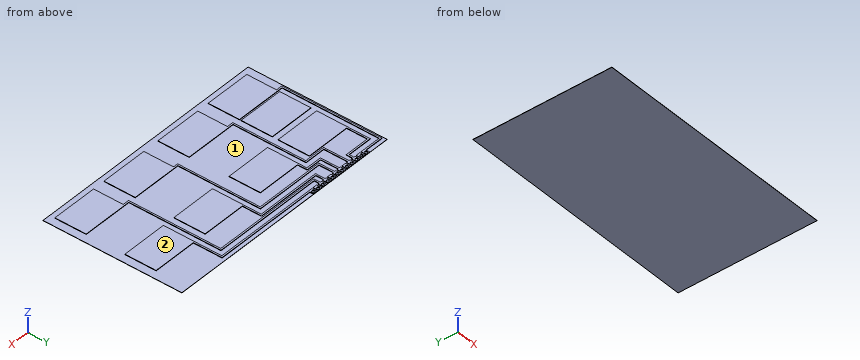
from build123d import *

# Parameters (mm, degrees)
F0_W     = 308
F0_H     = 174
F1_DEPTH = 0.25
F2_R     = 1.6
F2_W     = 57.88946
F2_H     = 39.180715
F3_DEPTH = 0.5


with BuildPart() as f1:
    # F0 (on Top) → F1 (new body)
    with BuildSketch(Plane.XY):
        Rectangle(F0_W, F0_H)
    extrude(amount=F1_DEPTH)

    # F2 (on face) → F3 (join)
    with BuildSketch(Plane.XY.offset(0.25)):
        Polygon((-86.945909, 80.4), (-86.945909, 87), (-92.145909, 87), (-92.145909, 80.4), (-90.545909, 80.4), (-88.545909, 80.4), align=None)
        with Locations((-89.545909, 84.5)):
            Circle(F2_R, mode=Mode.SUBTRACT)
        Polygon((-88.545909, 58.4), (-88.545909, 80.4), (-90.545909, 80.4), (-90.545909, 56.4), (-70.383385, 56.4), (-70.383385, 46.4), (-68.383385, 46.4), (-68.383385, 58.4), align=None)
        Polygon((-12.493925, 46.4), (-68.383385, 46.4), (-70.383385, 46.4), (-70.383385, 7.219285), (-12.493925, 7.219285), align=None)
        Polygon((-94.145909, 87), (-99.345909, 87), (-99.345909, 80.4), (-97.745909, 80.4), (-95.745909, 80.4), (-94.145909, 80.4), align=None)
        with Locations((-96.745909, 84.5)):
            Circle(F2_R, mode=Mode.SUBTRACT)
        Polygon((-101.345909, 87), (-106.545909, 87), (-106.545909, 80.4), (-104.945909, 80.4), (-102.945909, 80.4), (-101.345909, 80.4), align=None)
        with Locations((-103.945909, 84.5)):
            Circle(F2_R, mode=Mode.SUBTRACT)
        Polygon((-102.945909, 80.4), (-104.945909, 80.4), (-104.945909, 48.4), (-78.383385, 48.4), (-78.383385, -43.180715), (-70.383385, -43.180715), (-70.383385, -41.180715), (-76.383385, -41.180715), (-76.383385, 50.4), (-102.945909, 50.4), align=None)
        Polygon((-70.383385, -41.180715), (-70.383385, -43.180715), (-70.383385, -80.36143), (-10.637844, -80.36143), (-10.637844, -41.180715), align=None)
        Polygon((-108.545909, 87), (-113.745909, 87), (-113.745909, 80.4), (-112.145909, 80.4), (-110.145909, 80.4), (-108.545909, 80.4), align=None)
        with Locations((-111.145909, 84.5)):
            Circle(F2_R, mode=Mode.SUBTRACT)
        Polygon((-110.145909, 80.4), (-112.145909, 80.4), (-112.145909, 74.4), (-144, 74.4), (-144, 46.4), (-142, 46.4), (-142, 72.4), (-110.145909, 72.4), align=None)
        Polygon((-142, 46.4), (-144, 46.4), (-144, 7.219285), (-86.11054, 7.219285), (-86.11054, 46.4), align=None)
        Polygon((-115.745909, 87), (-120.945909, 87), (-120.945909, 80.4), (-119.345909, 80.4), (-117.345909, 80.4), (-115.745909, 80.4), align=None)
        with Locations((-118.345909, 84.5)):
            Circle(F2_R, mode=Mode.SUBTRACT)
        Polygon((-122.945909, 87), (-128.145909, 87), (-128.145909, 82.4), (-128.145909, 80.4), (-122.945909, 80.4), align=None)
        with Locations((-125.545909, 84.5)):
            Circle(F2_R, mode=Mode.SUBTRACT)
        Polygon((-128.145909, 80.4), (-128.145909, 82.4), (-152, 82.4), (-152, -43.180715), (-144, -43.180715), (-144, -41.180715), (-150, -41.180715), (-150, 80.4), align=None)
        Polygon((-144, -41.180715), (-144, -43.180715), (-144, -80.36143), (-86.11054, -80.36143), (-86.11054, -41.180715), align=None)
        Polygon((-81.345909, 80.4), (-79.745909, 80.4), (-79.745909, 87), (-84.945909, 87), (-84.945909, 80.4), (-83.345909, 80.4), align=None)
        with Locations((-82.345909, 84.5)):
            Circle(F2_R, mode=Mode.SUBTRACT)
        Polygon((-81.345909, 62.4), (-81.345909, 80.4), (-83.345909, 80.4), (-83.345909, 60.4), (4.493925, 60.4), (4.493925, -43.180715), (10.637844, -43.180715), (10.637844, -41.180715), (6.493925, -41.180715), (6.493925, 62.4), align=None)
        Polygon((70.383385, -41.180715), (10.637844, -41.180715), (10.637844, -43.180715), (10.637844, -80.36143), (70.383385, -80.36143), align=None)
        Polygon((-72.545909, 87), (-77.745909, 87), (-77.745909, 80.4), (-76.145909, 80.4), (-74.145909, 80.4), (-72.545909, 80.4), align=None)
        with Locations((-75.145909, 84.5)):
            Circle(F2_R, mode=Mode.SUBTRACT)
        Polygon((-65.345909, 87), (-70.545909, 87), (-70.545909, 80.4), (-68.945909, 80.4), (-66.945909, 80.4), (-65.345909, 80.4), align=None)
        with Locations((-67.945909, 84.5)):
            Circle(F2_R, mode=Mode.SUBTRACT)
        Polygon((-66.945909, 80.4), (-68.945909, 80.4), (-68.945909, 68.4), (12.493925, 68.4), (12.493925, 46.4), (14.493925, 46.4), (14.493925, 70.4), (-66.945909, 70.4), align=None)
        Polygon((14.493925, 46.4), (12.493925, 46.4), (12.493925, 7.219285), (70.383385, 7.219285), (70.383385, 46.4), align=None)
        Polygon((-58.145909, 87), (-63.345909, 87), (-63.345909, 80.4), (-61.745909, 80.4), (-59.745909, 80.4), (-58.145909, 80.4), align=None)
        with Locations((-60.745909, 84.5)):
            Circle(F2_R, mode=Mode.SUBTRACT)
        Polygon((-59.745909, 80.4), (-61.745909, 80.4), (-61.745909, 72.4), (78.11054, 72.4), (78.11054, -43.180715), (86.11054, -43.180715), (86.11054, -41.180715), (80.11054, -41.180715), (80.11054, 74.4), (-59.745909, 74.4), align=None)
        Polygon((86.11054, -41.180715), (86.11054, -43.180715), (86.11054, -80.36143), (144.087264, -80.36143), (144, -41.180715), align=None)
        Polygon((-50.945909, 87), (-56.145909, 87), (-56.145909, 80.4), (-54.545909, 80.4), (-52.545909, 80.4), (-50.945909, 80.4), align=None)
        with Locations((-53.545909, 84.5)):
            Circle(F2_R, mode=Mode.SUBTRACT)
        Polygon((-43.745909, 87), (-48.945909, 87), (-48.945909, 80.4), (-43.745909, 80.4), (-43.745909, 82.4), align=None)
        with Locations((-46.345909, 84.5)):
            Circle(F2_R, mode=Mode.SUBTRACT)
        Polygon((-43.745909, 82.4), (-43.745909, 80.4), (86.11054, 80.4), (86.11054, 46.4), (88.11054, 46.4), (88.11054, 82.4), align=None)
        Polygon((88.11054, 46.4), (86.11054, 46.4), (86.11054, 7.219285), (144, 7.219285), (144, 46.4), align=None)
        with Locations((-115.05527, -19.590357)):
            Rectangle(F2_W, F2_H)
    extrude(amount=F3_DEPTH)


solid = f1.part
Geometry check sheet. Reference: the model listing, model coordinates, mm. Face numbers are marked on the shaded views. Give positions to 0.01 mm unless a question says otherwise; leave off trailing zeros. Loops run counter-clockwise (first coordinate to the right, second up) from the corner with the lowest first, then second, coordinate; pieces in that order, holes last. Notation, with made-up numbers: M 31,-17.5 L 47,-17.5 A23 cw 47,18.5 Z; hole C 85,-9 d9. An arc over 180 degrees is marked long. Answer as a JSON object with one key per item and string values. Group by question number.
Item 1: Sectioned sample at C-C on y = -69.5. Record the boundary of the cut face in (x, z).
Item 2: Mould release check, pull along Y, two halves, no side actions. Record for the marked faces 1 and 2: pulls with the +Y half, pulls with the -Y half, needs draft (parallel to the pull), parting line crosses it, or undercut.
Item 3: Gauge pin test, flat end, axial feed: pin 1 (1 mm diameter, centred on x = 22.5, y = 63.5, fed in from +Z). Record the tip position at first contact, or that the pin passes through.
Item 4: Material ranges on L1, parallel to Y at x = -99, z = 0.5; L2, parallel to X at y = -64, z = 0.35; L3, parallel to Y at x = -18.5, z = 0.55, recorded low to high.
Item 5: Sectioned sample at B-B on z = 0.5. Give the number of separate pieces and of enclosed holes in the cut face, plus the area to 3 significant figures.
Item 6: Sectioned sample at A-A on x = -23. Record the boundary of the cut face in (y, z).
Findings below:
{
 "1": {"outline": "M -154,0 L 154,0 L 154,0.25 L 144.06,0.25 L 144.06,0.75 L 86.11,0.75 L 86.11,0.25 L 70.38,0.25 L 70.38,0.75 L 10.64,0.75 L 10.64,0.25 L -10.64,0.25 L -10.64,0.75 L -70.38,0.75 L -70.38,0.25 L -86.11,0.25 L -86.11,0.75 L -144,0.75 L -144,0.25 L -154,0.25 Z"},
 "2": {"face 1": "undercut", "face 2": "needs draft"},
 "3": {"pin 1": "z = 0.25"},
 "4": {"L1": "-80.36 to -41.18, -39.18 to 0, 7.22 to 46.4, 48.4 to 50.4, 80.4 to 87", "L2": "-144 to -86.11, -70.38 to -10.64, 10.64 to 70.38, 86.11 to 144.05", "L3": "-80.36 to -41.18, 7.22 to 46.4, 60.4 to 62.4, 68.4 to 70.4, 72.4 to 74.4, 80.4 to 82.4"},
 "5": {"separate pieces": "13", "enclosed holes": "12", "area": "23,300 mm2"},
 "6": {"outline": "M -87,0 L 87,0 L 87,0.25 L 82.4,0.25 L 82.4,0.75 L 80.4,0.75 L 80.4,0.25 L 74.4,0.25 L 74.4,0.75 L 72.4,0.75 L 72.4,0.25 L 70.4,0.25 L 70.4,0.75 L 68.4,0.75 L 68.4,0.25 L 62.4,0.25 L 62.4,0.75 L 60.4,0.75 L 60.4,0.25 L 46.4,0.25 L 46.4,0.75 L 7.22,0.75 L 7.22,0.25 L -41.18,0.25 L -41.18,0.75 L -80.36,0.75 L -80.36,0.25 L -87,0.25 Z"}
}
